Input: part model. Units: mm. Frame: model coordinates. A direction names the side the tool comes from. Give positions to 0.01 mm unless a question says otherwise; leave off trailing zeros. Write each loop counter-clockwise with the first axis right and the second up, starting at its lowest first coordinate (ties: lowest second). Pieces come first, ordered by that corner, then holes. Notation, with made-up numbers: (28, 14.25) - (78, 14.25) arc R31 cw to (78, 50.25) - close; hole circle Ø4 at (13, 1). An arc over 180 degrees is marked (long way). Answer as CSV lines item,"result".
```python
from build123d import *

# Parameters (mm, degrees)
F0_R     = 2.5
F1_DEPTH = 1.6
F2_R     = 3.45
F2_R_2   = 2.5
F3_DEPTH = 1.4


with BuildPart() as f1:
    # F0 (on Top) → F1 (new body)
    with BuildSketch(Plane.XY):
        with BuildLine():
            Line((-4, -7.5), (4, -7.5))
            ThreePointArc((4, -7.5), (4.707107, -7.207107), (5, -6.5))
            Line((5, -6.5), (5, 6.5))
            ThreePointArc((5, 6.5), (4.707107, 7.207107), (4, 7.5))
            Line((4, 7.5), (-4, 7.5))
            ThreePointArc((-4, 7.5), (-4.707107, 7.207107), (-5, 6.5))
            Line((-5, 6.5), (-5, -6.5))
            ThreePointArc((-5, -6.5), (-4.707107, -7.207107), (-4, -7.5))
        make_face()
        Circle(F0_R, mode=Mode.SUBTRACT)
    extrude(amount=F1_DEPTH)

    # F2 (on Top) → F3 (join)
    with BuildSketch(Plane.XY):
        Circle(F2_R)
        Circle(F2_R_2, mode=Mode.SUBTRACT)
    extrude(amount=-F3_DEPTH)


solid = f1.part
```
Item 1: Ray query, line 1 (Y direction, x = 0, z = 0.55); line 2 (Y direction, x = 0, z = -0.6); line 3 (Z direction, x = 2.5, y = -3.75). Return the intervals inside material, ascending. Write a range as from..to.
The answers:
line 1,"-7.5..-2.5, 2.5..7.5"
line 2,"-3.45..-2.5, 2.5..3.45"
line 3,"0..1.6"
Item 2: Contact query for a flat-ended pin moving along its axis: pin 1 (3 mm diameter, centred on x = 0, y = 0, fed in from -Z). Output: stop coordinate, or through.
The answers:
pin 1,"through"
Item 3: Reachability of faces 1 (the face through (4.699, -7.215, 0.789)), 2 (the face through (-1.2, 3.4, 0)) from +Z, -Z, +X, -X, +Y, -Y: full face, straight path, thin tool, end or side. Return the list, or none.
The answers:
face 1,"+Z, -Z, +X, -Y"
face 2,"-Z"
Item 4: Cut plane B-B on x = 0. Return the cut outline in (y, z), plus the area to 3 significant figures.
The answers:
outline,"(-7.5, 0) - (-3.45, 0) - (-3.45, -1.4) - (-2.5, -1.4) - (-2.5, 1.6) - (-7.5, 1.6) - close; (2.5, -1.4) - (3.45, -1.4) - (3.45, 0) - (7.5, 0) - (7.5, 1.6) - (2.5, 1.6) - close"
area,"18.7 mm²"
Item 5: Cut plane D-D on y = 3. Return the cut outline in (x, z).
The answers:
outline,"(-5, 0) - (-1.7, 0) - (-1.7, -1.4) - (1.7, -1.4) - (1.7, 0) - (5, 0) - (5, 1.6) - (-5, 1.6) - close"
Item 6: Cut plane C-C on z = 1.45. Return the cut outline in (x, y), plus the area to 3 significant figures.
The answers:
outline,"(-5, -6.5) arc R1 ccw to (-4, -7.5) - (4, -7.5) arc R1 ccw to (5, -6.5) - (5, 6.5) arc R1 ccw to (4, 7.5) - (-4, 7.5) arc R1 ccw to (-5, 6.5) - close; hole circle Ø5 at (0, 0)"
area,"130 mm²"
Item 7: Cut plane A-A on y = 0. Return the cut outline in (x, z).
The answers:
outline,"(-5, 0) - (-3.45, 0) - (-3.45, -1.4) - (-2.5, -1.4) - (-2.5, 1.6) - (-5, 1.6) - close; (2.5, -1.4) - (3.45, -1.4) - (3.45, 0) - (5, 0) - (5, 1.6) - (2.5, 1.6) - close"
